Autodesk Inventor part; units mm, degrees
ref_plane "YZ Plane" through (0, 0, 0) normal (1, 0, 0) x (0, 1, 0)
ref_plane "XZ Plane" through (0, 0, 0) normal (0, 1, 0) x (-1, 0, 0)
ref_plane "XY Plane" through (0, 0, 0) normal (0, 0, 1) x (1, 0, 0)
sketch "Sketch1" plane through (0, 0, 0) normal (0, 0, 1) x (1, 0, 0)
  line L0 (-12.2, -17.05) -> (12.2, -17.05)
  line L1 (12.2, -17.05) -> (12.2, 17.05)
  line L2 (12.2, 17.05) -> (-12.2, 17.05)
  line L3 (-12.2, 17.05) -> (-12.2, -17.05)
  line L4 (-12.2, -17.05) -> (12.2, 17.05) construction
  line L5 (12.2, -17.05) -> (-12.2, 17.05) construction
  circle A0 centre (-10, 14.92) radius 1.5
  circle A1 centre (10, 14.92) radius 1.5
  line L6 (-10, 14.92) -> (10, 14.92) construction
  circle A2 centre (-9, 9.05) radius 0.8
  circle A3 centre (-10, 9.05) radius 0.8
  circle A4 centre (9, 9.05) radius 0.8
  circle A5 centre (10, 9.05) radius 0.8
  line L7 (-9, 9.05) -> (9, 9.05) construction
  line L8 (-10, 9.05) -> (10, 9.05) construction
  point P0 (0, 0)
  point P1 (0, 9.05)
  point P2 (0, 14.92)
  point P3 (0, 0)
  point P4 (0, 0)
  dimension "d0" = 24.4
  dimension "d1" = 34.1
  dimension "d2" = 2.13
  dimension "d3" = 3
  dimension "d4" = 10
  dimension "d13" = 20
  dimension "d14" = 18
  dimension "d15" = 1.6
  dimension "d16" = 8
extrude "Extrusion1" add sketch "Sketch1" along normal mid plane 1.6
sketch "Sketch2" plane through (0, 0, -0.8) normal (0, 0, -1) x (-1, 0, 0)
  circle A0 centre (-10, 14.92) radius 1.5
  circle A1 centre (10, 14.92) radius 1.5
  line L0 (-12.2, -17.05) -> (12.2, -17.05)
  line L1 (12.2, -17.05) -> (12.2, 17.05)
  line L2 (12.2, 17.05) -> (-12.2, 17.05)
  line L3 (-12.2, 17.05) -> (-12.2, -17.05)
  line L4 (-10.16, -12.99) -> (10.16, -12.99)
  line L5 (10.16, -12.99) -> (10.16, -15.53)
  line L6 (10.16, -15.53) -> (-10.16, -15.53)
  line L7 (-10.16, -15.53) -> (-10.16, -12.99)
  point P0 (0, 0)
  point P1 (0, -12.99)
  point P2 (-10.16, -14.26)
  dimension "d8" = 2.54
  dimension "d9" = 20.32
  dimension "d10" = 2.79
extrude "Extrusion2" add sketch "Sketch2" along normal blind 2.5 contours L4 L5 L6 L7
sketch "Sketch3" plane through (0, 0, 0.8) normal (0, 0, 1) x (1, 0, 0)
  circle A0 centre (10, 14.92) radius 1.5
  circle A1 centre (-10, 14.92) radius 1.5
  arc A2 (-9.5, 8.4255) -> (-9.5, 9.6745) centre (-9, 9.05) ccw
  arc A3 (-9.5, 9.6745) -> (-9.5, 8.4255) centre (-10, 9.05) ccw
  line L0 (-12.2, -17.05) -> (12.2, -17.05)
  line L1 (12.2, -17.05) -> (12.2, 17.05)
  line L2 (12.2, 17.05) -> (-12.2, 17.05)
  line L3 (-12.2, 17.05) -> (-12.2, -17.05)
  arc A4 (9.5, 9.6745) -> (9.5, 8.4255) centre (9, 9.05) ccw
  arc A5 (9.5, 8.4255) -> (9.5, 9.6745) centre (10, 9.05) ccw
  line L4 (-3.4725, 12.5225) -> (3.4725, 12.5225)
  line L5 (3.4725, 12.5225) -> (3.4725, 5.5775)
  line L6 (3.4725, 5.5775) -> (-3.4725, 5.5775)
  line L7 (-3.4725, 5.5775) -> (-3.4725, 12.5225)
  point P0 (0, 0)
  point P1 (3.4725, 9.05)
  point P2 (0, 12.5225)
  dimension "d17" = 6.945
extrude "Extrusion3" add sketch "Sketch3" along normal blind 0.78 contours L4 L5 L6 L7
sketch "Sketch4" plane through (0, 0, 1.58) normal (0, 0, 1) x (1, 0, 0)
  line L0 (3.4725, 12.5225) -> (-3.4725, 12.5225)
  line L1 (-3.4725, 12.5225) -> (-3.4725, 5.5775)
  line L2 (-3.4725, 5.5775) -> (3.4725, 5.5775)
  line L3 (3.4725, 5.5775) -> (3.4725, 12.5225)
  circle A0 centre (0, 9.05) radius 3.175
  point P0 (0, 0)
  point P1 (0, 12.5225)
  point P2 (-3.4725, 9.05)
  dimension "d20" = 6.35
extrude "Extrusion4" cut sketch "Sketch4" against normal blind 0.1 contours A0
equation "\"d9\" = 8 * d8"
properties part number "Module_ArducamMini" material "Epoxy Resin"
The listing builds one solid part. Answer for the finished solid, in the listing's coordinates (mm). A direction names the side the tool comes from. Coordinates: 2 decimals unless noted, no trailing zeros. Loops run counter-clockwise (first coordinate to the right, second up) from the corner with the lowest first, then second, coordinate; pieces in that order, holes last.
1) A tool of negligible diameter and unlimited length cuts with its end or side. For faces 5 (the face through (0, -15.53, -2)), 6 (the face through (-10.16, -14, -2)), 7 (the face through (0, 9, 1.48)), 8 (the face through (10.16, -14, -2)), from which of +Z, -Z, +X, -X, +Y, -Y can it reach the whole face along a straight path? Write none if from no direction.
2) Find section C-C on x = -9. Write down the section's boundary in (y, z), then the cut area to 3 significant figures.
3) Find section D-D on z = 0.1. Write down the section's boundary in (x, y), then the cut area to 3 significant figures.
4) Find the intervals of material crossed by L1, parallel to Y at x = -10, z = 0.5; L2, parallel to Y at x = -9, z = -0.15; L3, parallel to Z at x = -5.25, y = 10, in increasing order.
5) Determine the mould class of faces 1 (the face through (-8.2, 9.1, 0)), 2 (the face through (0, 0, 0.8)), 3 (the face through (10.8, 9.1, 0)), 4 (the face through (0, 17.05, 0)) for opening direction Y: pulls with the +Y half, pulls with the -Y half, needs draft (parallel to the pull), parting line crosses it, or undercut.
6) Find section A-A on y = 9.05. Give the number of separate pieces and of enclosed holes in the cut face, then the cut area to 3 significant figures.
7) Flat-ended cylindrical pins translate along their axes: pin 1 Ø1.4 at (x, y) = (-9, 9.05) entering from +Z; pin 2 Ø0.8 at (x, z) = (-3.5, -2) entering from -Y; pin 3 Ø1.8 at (x, y) = (9, 9.05) entering from -Z; pin 4 Ø5 at (x, y) = (0, 9.05) entering from +Z. Find the tip coordinate at first contact, or state that the pin passes through.
Values:
1. face 5: -Z, +X, -X, -Y
1. face 6: -Z, -X, +Y, -Y
1. face 7: +Z
1. face 8: -Z, +X, +Y, -Y
2. outline: (-17.05, -0.8) - (-15.53, -0.8) - (-15.53, -3.3) - (-12.99, -3.3) - (-12.99, -0.8) - (8.25, -0.8) - (8.25, 0.8) - (-17.05, 0.8) - close; (9.85, -0.8) - (13.8, -0.8) - (13.8, 0.8) - (9.85, 0.8) - close; (16.04, -0.8) - (17.05, -0.8) - (17.05, 0.8) - (16.04, 0.8) - close
2. area: 54.8 mm2
3. outline: (-12.2, -17.05) - (12.2, -17.05) - (12.2, 17.05) - (-12.2, 17.05) - close; hole circle Ø3 at (-10, 14.92); hole (-9.5, 8.43) arc R0.8 ccw (long way) to (-9.5, 9.67) arc R0.8 ccw (long way) to start; hole circle Ø3 at (10, 14.92); hole (9.5, 8.43) arc R0.8 ccw (long way) to (9.5, 9.67) arc R0.8 ccw (long way) to start
3. area: 811 mm2
4. L1: y = -17.05 to 8.25, 9.85 to 13.42, 16.42 to 17.05
4. L2: y = -17.05 to 8.25, 9.85 to 13.8, 16.04 to 17.05
4. L3: z = -0.8 to 0.8
5. face 1: undercut
5. face 2: needs draft
5. face 3: undercut
5. face 4: pulls with the +Y half
6. separate pieces: 3
6. enclosed holes: 0
6. area: 35.5 mm2
7. pin 1: passes through
7. pin 2: stops at y = -15.53
7. pin 3: stops at z = -0.8
7. pin 4: stops at z = 1.48
